Print and shaded views of the part. All mm, measured from the part's lowest x, y and z. A direction names the side the tool comes from. Coordinates: 2 decimals unless noted, no trailing zeros. Order: outer loops, then holes, each group sorted by start corner. A loop starts at its lowest first (then second) coordinate and runs counter-clockwise, first axis right, second up. Notation, with made-up numbers: (13, -27.75) - (63, -27.75) arc R9 ccw to (63, -16.75) - close; hole circle Ø5 at (-17.75, -17). An arc over 180 degrees is marked (long way). Write each question's results on one line, items separated by ' | '.
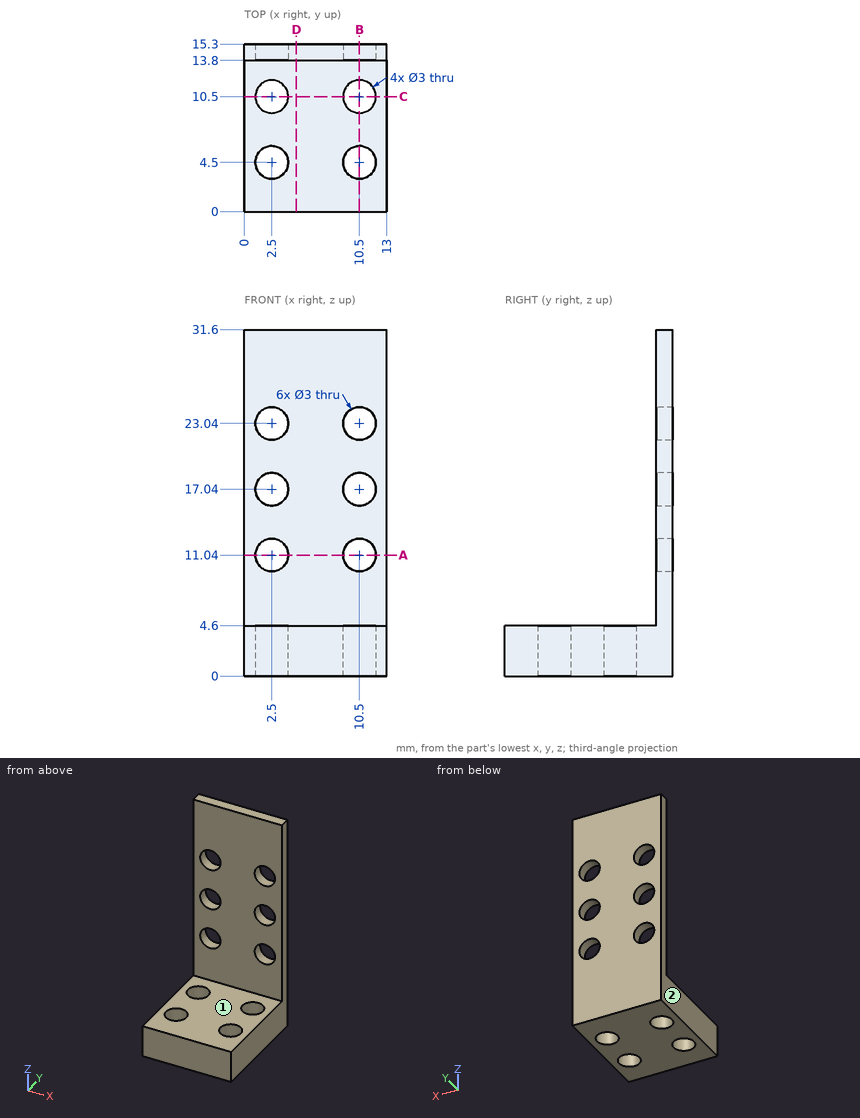
1. Band-saw the part on D-D on x = 4.75. Give the cut face in (y, z).
Solved:
outline: (0, 0) - (15.3, 0) - (15.3, 31.6) - (13.8, 31.6) - (13.8, 4.6) - (0, 4.6) - close
2. Drop flat-ended pins along their axis: pin 1 Ø6 at (y, z) = (10, 20) entering from +X; pin 2 Ø4 at (x, y) = (3, 1.5) entering from +Z; pin 3 Ø4 at (x, z) = (2.5, 23.04) entering from -Y. Give the stop position or say it passes through.
Solved:
pin 1: passes through | pin 2: stops at z = 4.6 | pin 3: stops at y = 13.8
3. Band-saw the part on A-A on z = 11.04. Give the cut face in (x, y).
Solved:
outline: (0, 13.8) - (1, 13.8) - (1, 15.3) - (0, 15.3) - close; (4, 13.8) - (9, 13.8) - (9, 15.3) - (4, 15.3) - close; (12, 13.8) - (13, 13.8) - (13, 15.3) - (12, 15.3) - close
4. Tool access for the marked faces 1 and 2: list every direction of +Z, -Z, +X, -X, +Y, -Y with a clear straight run to the whole face (end or side of a thin tool).
Solved:
face 1: +Z, +X, -X, -Y | face 2: +Z, -Z, -X, +Y, -Y
5. Probe line 1 (X direction, y = 14.95, z = 23.04); line 2 (Z direction, x = 10.5, y = 14.5); line 3 (Y direction, x = 3, z = 2.5). List the from-to ranges inside material, lowest first.
Solved:
line 1: x = 0 to 1, 4 to 9, 12 to 13 | line 2: z = 0 to 9.54, 12.54 to 15.54, 18.54 to 21.54, 24.54 to 31.6 | line 3: y = 0 to 3.09, 5.91 to 9.09, 11.91 to 15.3
6. Band-saw the part on C-C on y = 10.5. Give the cut face in (x, z), then the cut area to 3 significant figures.
Solved:
outline: (0, 0) - (1, 0) - (1, 4.6) - (0, 4.6) - close; (4, 0) - (9, 0) - (9, 4.6) - (4, 4.6) - close; (12, 0) - (13, 0) - (13, 4.6) - (12, 4.6) - close | area: 32.2 mm2
7. Band-saw the part on B-B on x = 10.5. Give the cut face in (y, z).
Solved:
outline: (0, 0) - (3, 0) - (3, 4.6) - (0, 4.6) - close; (6, 0) - (9, 0) - (9, 4.6) - (6, 4.6) - close; (12, 0) - (15.3, 0) - (15.3, 9.54) - (13.8, 9.54) - (13.8, 4.6) - (12, 4.6) - close; (13.8, 12.54) - (15.3, 12.54) - (15.3, 15.54) - (13.8, 15.54) - close; (13.8, 18.54) - (15.3, 18.54) - (15.3, 21.54) - (13.8, 21.54) - close; (13.8, 24.54) - (15.3, 24.54) - (15.3, 31.6) - (13.8, 31.6) - close
